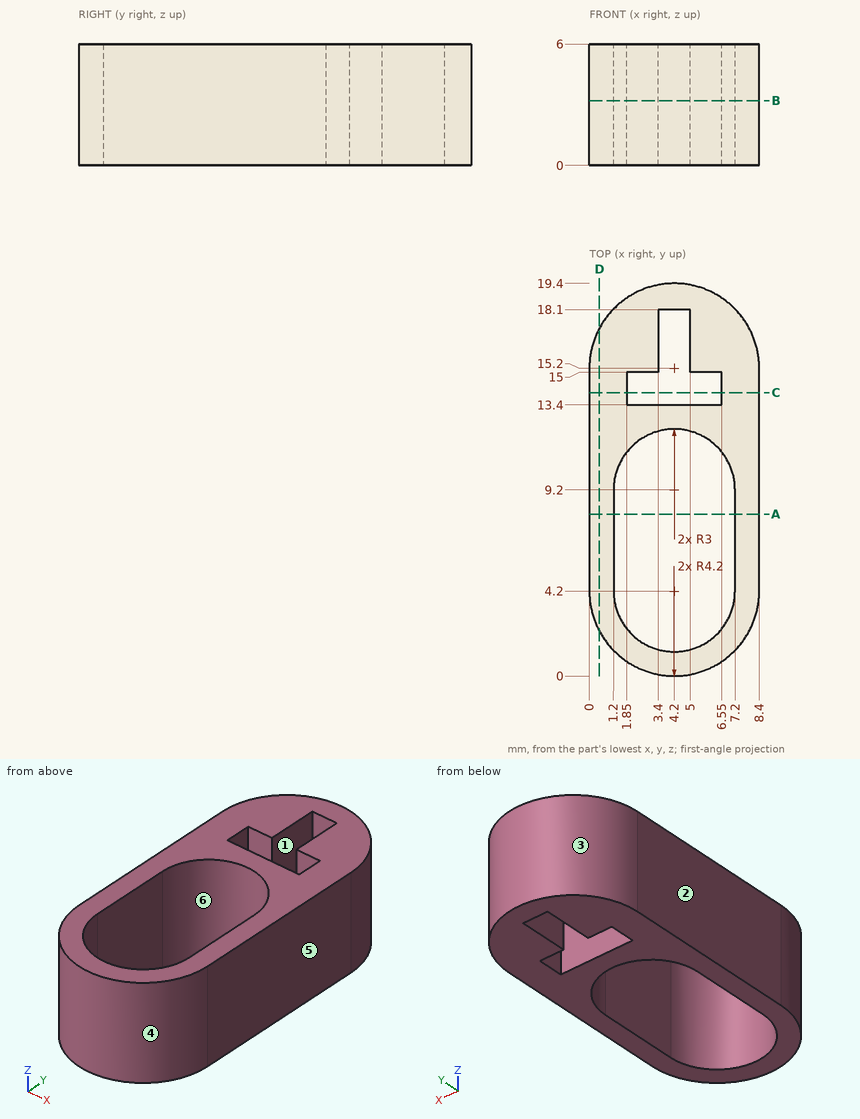
The figure shows three views and two pictorial views of one solid part (mm, origin at its lowest corner). Answer the questions. A direction names the side the tool comes from. Coordinates: 2 decimals unless noted, no trailing zeros. Loops run counter-clockwise (first coordinate to the right, second up) from the corner with the lowest first, then second, coordinate; pieces in that order, holes last.
1) Flat-ended cylindrical pins translate along their axes: pin 1 Ø1 at (y, z) = (3, 5.5) entering from -X; pin 2 Ø2 at (x, z) = (6, 2) entering from +Y; pin 3 Ø0.5 at (x, z) = (5.5, 3) entering from -Y. Find the tip coordinate at first contact, or state that the pin passes through.
2) Find section A-A on y = 8. Write down the section's boundary in (x, z), then the cut area to 3 significant figures.
3) Find section B-B on z = 3.2. Write down the section's boundary in (x, y), then the cut area to 3 significant figures.
4) Find section C-C on y = 14. Write down the section's boundary in (x, z), then the cut area to 3 significant figures.
5) Find section D-D on x = 0.5. Write down the section's boundary in (y, z).
6) Determine the mould class of the marked faces 3, 4, 5 and 6 for opening direction Y: pulls with the +Y half, pulls with the -Y half, needs draft (parallel to the pull), parting line crosses it, or undercut.
7) A tool of negligible diameter and unlimited length cuts with its end or side. For the marked faces 1 and 2, from which of +Z, -Z, +X, -X, +Y, -Y can it reach the whole face along a straight path? Write none if from no direction.
8) Find the intervals of material crossed by L1, parallel to X at y = 14.75, z = 1.3; L2, parallel to Y at x = 4.5, z = 2; L3, parallel to Y at x = 6.25, z = 5.7, in increasing order.
Values:
1. pin 1: stops at x = 0.06
1. pin 2: stops at y = 19.32
1. pin 3: stops at y = 0.13
2. outline: (0, 0) - (1.2, 0) - (1.2, 6) - (0, 6) - close; (7.2, 0) - (8.4, 0) - (8.4, 6) - (7.2, 6) - close
2. area: 14.4 mm2
3. outline: (0, 4.2) arc R4.2 ccw to (8.4, 4.2) - (8.4, 15.2) arc R4.2 ccw to (0, 15.2) - close; hole (1.2, 4.2) arc R3 ccw to (7.2, 4.2) - (7.2, 9.2) arc R3 ccw to (1.2, 9.2) - close; hole (1.85, 13.4) - (6.55, 13.4) - (6.55, 15) - (5, 15) - (5, 18.1) - (3.4, 18.1) - (3.4, 15) - (1.85, 15) - close
3. area: 77.1 mm2
4. outline: (0, 0) - (1.85, 0) - (1.85, 6) - (0, 6) - close; (6.55, 0) - (8.4, 0) - (8.4, 6) - (6.55, 6) - close
4. area: 22.2 mm2
5. outline: (2.21, 0) - (17.19, 0) - (17.19, 6) - (2.21, 6) - close
6. face 3: pulls with the +Y half
6. face 4: pulls with the -Y half
6. face 5: needs draft
6. face 6: undercut
7. face 1: +Z, -Z
7. face 2: +Z, -Z, -X, +Y, -Y
8. L1: x = 0 to 1.85, 6.55 to 8.4
8. L2: y = 0.01 to 1.22, 12.18 to 13.4, 18.1 to 19.39
8. L3: y = 0.53 to 2.01, 11.39 to 13.4, 15 to 18.87
